Can you work these out from the model? Positions are in its coordinate system, mm. A direction names the side the tool comes from. Round coordinates to 2 decimals unless told otherwise and drop trailing zeros. Loops run counter-clockwise (first coordinate to the right, second up) from the corner with the lowest first, then second, coordinate; pieces in that order, holes last. Notation, with made-up numbers: (-40, 20.25) -> (-13, 20.25) arc R17 ccw to (-13, 34.25) -> close; hole circle Ø10 at (22, 3.25). An arc over 180 degrees is marked (long way). Write item = value, one per line.
from build123d import *

# Parameters (mm, degrees)
SKETCH1_W                  = 31.75
SKETCH1_H                  = 25.4
BOSS_EXTRUDE1_DEPTH        = 9.525
M2_5_CLEARANCE_HOLE1_D     = 3.1
M2_5_CLEARANCE_HOLE1_DEPTH = 8.001
M2_5_CLEARANCE_HOLE1_TIP   = 0.931333959
SKETCH3_W                  = 9.525
SKETCH3_H                  = 19.942491079
BOSS_EXTRUDE2_DEPTH        = 25.4
F_4_CLEARANCE_HOLE1_D      = 3.4544
SKETCH9_W                  = 5.8975
SKETCH9_H                  = 5.8975
CUT_EXTRUDE1_DEPTH         = 1.09455
SKETCH10_W                 = 5.453
SKETCH10_H                 = 6.0499
CUT_EXTRUDE2_DEPTH         = 1.1771


with BuildPart() as part:
    # Sketch1 → Boss-Extrude1 (new body)
    with BuildSketch(Plane(origin=(0, 0, 0), x_dir=(1, 0, 0), z_dir=(0, 1, 0))):
        Rectangle(SKETCH1_W, SKETCH1_H)
    extrude(amount=BOSS_EXTRUDE1_DEPTH)

    # M2.5 Clearance Hole1
    with Locations(Plane(origin=(8, 0, -8), x_dir=(0, 0, -1), z_dir=(0, -1, 0))):
        with Locations((0, 0), (-16, 0), (-16, -16), (0, -16)):
            Hole(M2_5_CLEARANCE_HOLE1_D / 2, depth=M2_5_CLEARANCE_HOLE1_DEPTH)
            with Locations((0, 0, -(M2_5_CLEARANCE_HOLE1_DEPTH + M2_5_CLEARANCE_HOLE1_TIP / 2))):  # 118° drill point
                Cone(0, M2_5_CLEARANCE_HOLE1_D / 2, M2_5_CLEARANCE_HOLE1_TIP, mode=Mode.SUBTRACT)

    # Sketch3 → Boss-Extrude2 (add)
    with BuildSketch(Plane(origin=(0, 0, -12.7), x_dir=(-1, 0, 0), z_dir=(0, 0, -1))):
        with Locations((11.1379, 19.49624554)):
            Rectangle(SKETCH3_W, SKETCH3_H)
        with Locations((-11.1379, 19.49624554)):
            Rectangle(SKETCH3_W, SKETCH3_H)
    extrude(amount=-BOSS_EXTRUDE2_DEPTH)

    # #4 Clearance Hole1 (through all)
    with Locations(Plane(origin=(15.9004, 0, 0), x_dir=(0, 0, -1), z_dir=(1, 0, 0))):
        with Locations((0, 15.08125), (6.35, 23.8125), (-6.35, 23.8125)):
            Hole(F_4_CLEARANCE_HOLE1_D / 2)

    # Sketch9 → Cut-Extrude1 (cut, symmetric)
    with BuildSketch(Plane(origin=(11.1379, 0, 0), x_dir=(0, 0, -1), z_dir=(1, 0, 0))):
        with Locations((6.35, 23.8125)):
            Rectangle(SKETCH9_W, SKETCH9_H)
        with Locations((0, 15.08125)):
            Rectangle(SKETCH9_W, SKETCH9_H)
        with Locations((-6.35, 23.8125)):
            Rectangle(SKETCH9_W, SKETCH9_H)
    extrude(amount=CUT_EXTRUDE1_DEPTH, both=True, mode=Mode.SUBTRACT)

    # Sketch10 → Cut-Extrude2 (cut, symmetric)
    with BuildSketch(Plane(origin=(0, 4.7625, 0), x_dir=(-1, 0, 0), z_dir=(0, -1, 0))):
        with Locations((-8, 8)):
            Rectangle(SKETCH10_W, SKETCH10_H)
        with Locations((8, 8)):
            Rectangle(SKETCH10_W, SKETCH10_H)
        with Locations((8, -8)):
            Rectangle(SKETCH10_W, SKETCH10_H)
        with Locations((-8, -8)):
            Rectangle(SKETCH10_W, SKETCH10_H)
    extrude(amount=CUT_EXTRUDE2_DEPTH, both=True, mode=Mode.SUBTRACT)


solid = part.part
1. Suppose I cut it at D-D, the plane x = 13.5. List the corners of the cut face in (y, z) for me, and give its area (3 significant figures).
Entries:
outline = (0, -12.7) -> (29.47, -12.7) -> (29.47, 12.7) -> (0, 12.7) -> close; hole circle Ø3.45 at (15.08, 0); hole circle Ø3.45 at (23.81, -6.35); hole circle Ø3.45 at (23.81, 6.35)
area = 720 mm²
2. For faces 5 (the flat face through (-6.375, 19, 0)), 6 (the cylindrical face through (8.18, 25.27, -5.42)), 7 (the flat face through (10.043, 25, -8)), which set-ups out of +Z, -Z, +X, -X, +Y, -Y let a thin tool reach every point of the face, with its end or its side?
Entries:
face_5 = +Z, -Z, +Y
face_6 = +X, -X
face_7 = none
3. I need wall thicknesses on line 1 (Z direction, x = -8, y = 6.55); line 2 (X direction, y = 1.4, z = 8) (3 decimals); line 3 (Y direction, x = -10, z = 6.5). Which ranges of each line are inside material? Lowest first, please. Write a range as [from, to].
Entries:
line_1 = [-12.7, -9.55], [-6.45, 6.45], [9.55, 12.7]
line_2 = [-15.875, -9.55], [-6.45, 6.45], [9.55, 15.875]
line_3 = [0, 3.59], [5.94, 22.09], [25.53, 29.47]
4. I'm going to push flat-ended pins straight in: pin 1 (1.8 mm diameter, centred on y = 25, z = 5.5, fed in from +X); pin 2 (1.9 mm diameter, centred on x = 8, z = -8, fed in from -Y); pin 3 (2.5 mm diameter, centred on y = 5.5, z = 8, fed in from -X) (3 decimals); pin 4 (3 mm diameter, centred on x = -8, z = 8, fed in from -Y). Where does each tip first touch, or does it pass through?
Entries:
pin_1 = 15.9
pin_2 = 8.36
pin_3 = -15.875
pin_4 = 8.03
5. Suppose I cut it at A-A, the plane z = 0. Count the separate pieces of the cut face and the enclosed holes in it, and give its area (3 significant figures).
Entries:
separate_pieces = 3
enclosed_holes = 0
area = 611 mm²
6. We'd pull the mould along X, two halves only. Please class faces 1 (the flat face through (5.274, 5, 8)), 2 (the flat face through (15.9, 19, 0)), 3 (the cylindrical face through (-11.2, 13.4, -0.4)), 4 (the flat face through (11, 20.864, -6)): released by +X, released by -X, zero draft, split by the parting line, or undercut.
Entries:
face_1 = undercut
face_2 = released by +X
face_3 = zero draft
face_4 = undercut
7. Suppose I cut it at C-C, the plane y = 4.25. List the corners of the cut face in (x, z) for me (1 decimal), and give its area (3 significant figures).
Entries:
outline = (-15.9, -12.7) -> (15.9, -12.7) -> (15.9, 12.7) -> (-15.9, 12.7) -> close; hole (-10.7, -11) -> (-5.3, -11) -> (-5.3, -5) -> (-10.7, -5) -> close; hole (-10.7, 5) -> (-5.3, 5) -> (-5.3, 11) -> (-10.7, 11) -> close; hole (5.3, -11) -> (10.7, -11) -> (10.7, -5) -> (5.3, -5) -> close; hole (5.3, 5) -> (10.7, 5) -> (10.7, 11) -> (5.3, 11) -> close
area = 674 mm²
